Autodesk Inventor part; units mm, degrees
ref_plane "YZ Plane" through (0, 0, 0) normal (1, 0, 0) x (0, 1, 0)
ref_plane "XZ Plane" through (0, 0, 0) normal (0, 1, 0) x (-1, 0, 0)
ref_plane "XY Plane" through (0, 0, 0) normal (0, 0, 1) x (1, 0, 0)
sketch "Skizze1" plane through (0, 0, 0) normal (0, 1, 0) x (-1, 0, 0)
  circle A0 centre (0, 0) radius 30
  circle A1 centre (0, 0) radius 7
  line L0 (7, 0) -> (30, 0)
  line L1 (-7, 0) -> (-30, 0)
  line L2 (42, 0) -> (-42, 0)
  line L3 (0, -42) -> (0, 42)
  dimension "d0" = 60
  dimension "d1" = 14
  dimension "d2" = 0
extrude "Extrusion1" add sketch "Skizze1" along normal blind 3 contours L0 A1 L3 A0 | L3 A1 L1 A0 picked at (15.508, 15.8775) picked at (-21.0338, 7.0833)
sketch "Skizze3" plane through (0, 3, 0) normal (0, 1, 0) x (1, 0, 0)
  circle A0 centre (0, 0) radius 7.9
  circle A1 centre (0, 0) radius 7
  arc A2 (-7, 0) -> (7, 0) centre (0, 0) ccw
  line L0 (30, 0) -> (7, 0)
  line L1 (7.9, 0) -> (-7.9, 0)
  dimension "d13" = 15.8
extrude "Extrusion3" add sketch "Skizze3" along normal blind 15 contours A0 L1 A1 L0 picked at (7.5235, -0.6302)
sketch "Skizze4" plane through (-7, 0, 0) normal (0, 0, -1) x (-1, 0, 0)
  circle A0 centre (-186.9335, 0) radius 209.9335
  line L0 (106.9734, 0) -> (-480.8404, 0)
  line L1 (-7, -293.9069) -> (-7, 293.9069)
  line L2 (23, 0) -> (23, 3)
  circle A1 centre (-186.9335, 0) radius 191.832
  circle A2 centre (-186.9335, 0) radius 168.168
  circle A3 centre (-186.9335, 0) radius 150.0665
  line L3 (-39.8962, -30) -> (20.8454, -30)
  line L4 (2.5382, -30) -> (20.8454, -30)
  line L5 (-21.463, -30) -> (-39.8962, -30)
  point P0 (-7, 0)
  point P1 (4.8985, 0)
  point P2 (-18.7655, 0)
  point P3 (-36.867, 0)
  dimension "d16" = 419.867
  dimension "d17" = 383.664
  dimension "d18" = 336.336
  dimension "d19" = 300.133
  dimension "d20" = 30
extrude "Extrusion4" add sketch "Skizze4" against normal blind 5 contours L3 A1 L0 A0 | L3 A3 L0 A2 picked at (-33.1917, -26.6918)
sketch "Skizze5" plane through (-7.9, 3, 0) normal (0, 0, -1) x (-1, 0, 0)
  circle A0 centre (-187.8335, -3) radius 209.9335
  line L0 (22.1, -3) -> (22.1, 0)
  circle A1 centre (-187.8335, -3) radius 191.832
  circle A2 centre (-187.8335, -3) radius 168.168
  circle A3 centre (-187.8335, -3) radius 150.0665
  arc A4 (19.9454, -33) -> (22.1, -3) centre (-187.8335, -3) ccw
  line L1 (1.6382, -33) -> (19.9454, -33)
  line L2 (19.9454, -33) -> (1.6382, -33)
  line L3 (1.6382, -33) -> (-22.363, -33)
  line L4 (-40.7962, -33) -> (-22.363, -33)
  line L5 (22.1, -3) -> (3.9985, -3)
  line L6 (21.6804, -3) -> (-37.4804, -3)
  line L7 (-19.6655, -3) -> (-37.767, -3)
  point P0 (-7.9, -3)
  point P1 (193.7355, 3.1959)
  point P2 (175.634, 3.1959)
  point P3 (151.97, 3.1959)
  point P4 (133.8685, 3.1959)
  point P5 (19.9454, -33)
  dimension "d23" = 419.867
  dimension "d24" = 383.664
  dimension "d25" = 336.336
  dimension "d26" = 300.133
extrude "Extrusion5" cut sketch "Skizze5" against normal blind 2 contours A0 L1 A1 L5 | L4 A3 L7 L6 A2 picked at (8.1773, -29.6819) picked at (-34.0917, -29.6918)
sketch "Skizze6" plane through (-7, 0, 5) normal (0, 0, 1) x (1, 0, 0)
  line L0 (36.5804, 0) -> (-22.5804, 0)
  line L1 (-23, 0) -> (-23, 3)
  circle A0 centre (186.9335, 0) radius 200.8827
  arc A1 (-23, 0) -> (-20.8454, -30) centre (186.9335, 0) ccw
  circle A2 centre (186.9335, 0) radius 159.1173
  point P0 (7, 0)
  point P1 (-13.3884, -15)
  point P2 (28.5249, -15)
  dimension "d32" = 401.7655
  dimension "d33" = 318.2345
  dimension "d30" = 15
  dimension "d34" = 15
hole "Bohrung1" at (-20.3884, -15, 5) at (21.5249, -15, 5) direction (0, 0, -1) diameter 4 depth 10 tip angle 118
properties part number "Verbindungsstück-rechts-15mm-Ph-L"
Here's how the part is built. I have some questions about the finished solid (model axes, mm). A direction names the side the tool comes from. Coordinates: 2 decimals unless noted, no trailing zeros. Order: outer loops, then holes, each group sorted by start corner. A loop starts at its lowest first (then second) coordinate and runs counter-clockwise, first axis right, second up. Notation, with made-up numbers: (48, 50.5) - (102, 50.5) arc R21 cw to (102, 70.5) - close; hole circle Ø1 at (82.5, 75). An arc over 180 degrees is marked (long way). Use CSV: the item, a comma, the result in double quotes. Start each with the question number.
1. For faces 1 (the face through (25, -15, 5)), 2 (the face through (0.17, 10.4, 7.9)), 3 (the face through (-17, -15, 2)), which set-ups out of +Z, -Z, +X, -X, +Y, -Y let a thin tool reach every point of the face, with its end or its side?
2. I'm going to push flat-ended pins straight in: pin 1 (10.5 mm diameter, centred on x = 25.5, y = -20, fed in from -Z); pin 2 (5 mm diameter, centred on y = 3.5, z = 13, fed in from -X); pin 3 (8 mm diameter, centred on y = -20.5, z = 4, fed in from -X). Where does each tip first touch, or does it pass through?
3. Suppose I cut it at C-C on z = 6. List the corners of the cut face in (x, y) for me.
4. Please list where these lines run through material, in increasing order: line 1 (X direction, y = -15, z = 2.9); line 2 (Z direction, x = -14, y = -23.5); line 3 (X direction, y = 11, z = 1.5). Write a range as from..to.
5. Suppose I cut it at D-D on x = 0. List the corners of the cut face in (y, z) for me, then the cut area to 3 significant figures.
6. Suppose I cut it at B-B on y = -15. List the corners of the cut face in (x, z) for me.
7. If we mould it in two halves opening along Y, with no side actions, what happens to faces 4 (the face through (-17, -15, 5)), 5 (the face through (-18.436, -14.566, 3.479)), 6 (the face through (12.46, -15.27, 3.48))? For each: +Y half, -Y half, draft (parallel to the pull), parting line (faces both ways), or undercut.
8. Suppose I cut it at A-A on y = -21. List the corners of the cut face in (x, z) for me, then the cut area to 3 significant figures.
Output:
1,face 1,"+Z, +X, -X, -Y"
1,face 2,"+Z, +Y"
1,face 3,"-Z, +X, -X, -Y"
2,pin 1,"stops at z = 2"
2,pin 2,"stops at x = -28.08"
2,pin 3,"stops at x = -29.35"
3,outline,"(-29.39, 0) - (-3.61, 0) - (-3.61, 18) - (-5.14, 18) - (-5.14, 3) - (-29.39, 3) - close; (3.61, 0) - (29.39, 0) - (29.39, 3) - (5.14, 3) - (5.14, 18) - (3.61, 18) - close"
4,line 1,"x = -29.46..-22.39, -18.39..-11.31, 12.44..19.52, 23.52..30.62"
4,line 2,"z = 2..5"
4,line 3,"x = -7.76..-6.84, 6.84..7.76"
5,outline,"(0, 7) - (18, 7) - (18, 7.9) - (3, 7.9) - (3, 30) - (0, 30) - close"
5,area,"82.5 mm2"
6,outline,"(-29.46, 2) - (-22.39, 2) - (-22.39, 5) - (-29.46, 5) - close; (-18.39, 2) - (-11.31, 2) - (-11.31, 5) - (-18.39, 5) - close; (12.44, 2) - (19.52, 2) - (19.52, 5) - (12.44, 5) - close; (23.52, 2) - (30.62, 2) - (30.62, 5) - (23.52, 5) - close"
7,face 4,"draft"
7,face 5,"undercut"
7,face 6,"-Y half"
8,outline,"(-28.95, 2) - (-10.75, 2) - (-10.75, 5) - (-28.95, 5) - close; (13.08, 2) - (31.34, 2) - (31.34, 5) - (13.08, 5) - close"
8,area,"109 mm2"
